Here's how the part is built. I have some questions about the finished solid (model axes, mm). A direction names the side the tool comes from. Round coordinates to 2 decimals unless told otherwise and drop trailing zeros. Write each loop counter-clockwise with the first axis right and the second up, starting at its lowest first coordinate (ties: lowest second). Pieces come first, ordered by that corner, then holes. Notation, with made-up numbers: (53.5, 57.5) - (82.5, 57.5) arc R16 cw to (82.5, 77.5) - close; hole circle Ø7 at (-30, 37). An arc over 180 degrees is marked (long way). Write item = value, one per line. Start each with the question number.
Item 1: For P1, Ø7.5, axis at x = -18.12, z = -32.26, coming from the -Y side; P2, Ø7.5, axis at x = -37, z = -0.43, coming from the +Y side, each with a flat end and sliding along its axis, tell me the tip position at first contact or that it passes through.
Item 2: If we section it at D-D (y = -17.25): Please give me the cut outline in (x, z), and give its area (3 significant figures).
Item 3: If we section it at C-C (y = -2.25): Please give me the cut outline in (x, z), and give its area (3 significant figures).
Item 4: If we section it at A-A (x = 0): Please give me the cut outline in (y, z), and give its area (3 significant figures).
Item 5: Which directions (+Z, -Z, +X, -X, +Y, -Y) give clear straight access to the entire face, cutting with the end or side of a thin tool? Please do faces 4 (the face through (-18.75, -2.46, 34.62)), 5 (the face through (-10, -15, -51)), 6 (the face through (6, 0, 32)).
Item 6: If we section it at B-B (z = 0): Please give me the cut outline in (x, y), and give its area (3 significant figures).
Item 7: Thinking about a two-plate mould opening in Z: for faces 1 (the face through (-28, -5, 16)), 2 (the face through (-2, -5, -60)), 3 (the face through (0, -10, -51)), which applies, pulls with the +Z half, pulls with the -Z half, needs draft (parallel to the pull), parting line crosses it, or undercut?
Item 8: If I drill on line 1 along X through (y, z) = (-3.7, 0); line 2 along X through (y, z) = (-12, 0); line 3 along X through (y, z) = (2.5, 0), over which ranges is the centre line in solid material (lowest first)? Write a range as [from, to].
```python
from build123d import *

# Parameters (mm, degrees)
SKETCH1_W               = 220
SKETCH1_H               = 120
SKETCH1_R               = 43
BOSS_EXTRUDE1_DEPTH     = 10
SKETCH2_W               = 220
SKETCH2_H               = 120
SKETCH2_R               = 2.8
BOSS_EXTRUDE2_DEPTH     = 20
CUT_EXTRUDE1_REACH      = 166.012
CUT_EXTRUDE1_END_RADIUS = 43
SKETCH3_W               = 35
SKETCH3_H               = 10
SKETCH4_R               = 32
CUT_EXTRUDE2_DEPTH      = 127.885775404
CUT_EXTRUDE3_REACH      = 166.012
CUT_EXTRUDE3_END_RADIUS = 32
SKETCH5_W               = 20
SKETCH5_H               = 10
SKETCH6_R               = 42.5
CUT_EXTRUDE4_DEPTH      = 15


with BuildPart() as part:
    # Sketch1 → Boss-Extrude1 (new body)
    with BuildSketch(Plane(origin=(0, 0, 0), x_dir=(1, 0, 0), z_dir=(0, 1, 0))):
        Rectangle(SKETCH1_W, SKETCH1_H)
        with Locations(Location((0, 0, 0), (0, 0, 270))):
            Circle(SKETCH1_R, mode=Mode.SUBTRACT)
    extrude(amount=BOSS_EXTRUDE1_DEPTH)

    # Sketch2 → Boss-Extrude2 (add)
    with BuildSketch(Plane.XZ):
        Rectangle(SKETCH2_W, SKETCH2_H)
        with Locations(Location((18.122136771, 32.25814872, 0), (0, 0, 270))):
            Circle(SKETCH2_R, mode=Mode.SUBTRACT)
        with Locations(Location((36.997444656, 0.434843546, 0), (0, 0, 270))):
            Circle(SKETCH2_R, mode=Mode.SUBTRACT)
        with Locations(Location((18.875307886, -31.823305174, 0), (0, 0, 270))):
            Circle(SKETCH2_R, mode=Mode.SUBTRACT)
        with Locations(Location((-18.122136771, -32.25814872, 0), (0, 0, 270))):
            Circle(SKETCH2_R, mode=Mode.SUBTRACT)
        with Locations(Location((-36.997444656, -0.434843546, 0), (0, 0, 270))):
            Circle(SKETCH2_R, mode=Mode.SUBTRACT)
        with Locations(Location((-18.875307886, 31.823305174, 0), (0, 0, 270))):
            Circle(SKETCH2_R, mode=Mode.SUBTRACT)
    extrude(amount=BOSS_EXTRUDE2_DEPTH)

    # Cut-Extrude1: up to this cylinder (the profile starts outside it)
    cut_extrude1_end = Plane(origin=(0, 5, 0), z_dir=(0, -1, 0)) * Cylinder(CUT_EXTRUDE1_END_RADIUS, 419.024, mode=Mode.PRIVATE)
    # Sketch3 → Cut-Extrude1 (cut, up to the surface)
    with BuildSketch(Plane.XY.offset(60), mode=Mode.PRIVATE) as cut_extrude1_sk1:
        with Locations((0, 5)):
            Rectangle(SKETCH3_W, SKETCH3_H)
    cut_extrude1_tool1 = extrude(cut_extrude1_sk1.sketch, amount=-CUT_EXTRUDE1_REACH, mode=Mode.PRIVATE) - cut_extrude1_end
    add(cut_extrude1_tool1.solids().sort_by_distance((0, 5, 60))[0], mode=Mode.SUBTRACT)

    # Sketch4 → Cut-Extrude2 (cut, through all)
    with BuildSketch(Plane(origin=(0, 0, 0), x_dir=(1, 0, 0), z_dir=(0, 1, 0))):
        with Locations(Location((0, 0, 0), (0, 0, 270))):
            Circle(SKETCH4_R)
    extrude(amount=-CUT_EXTRUDE2_DEPTH, mode=Mode.SUBTRACT)

    # Cut-Extrude3: up to this cylinder (the profile starts outside it)
    cut_extrude3_end = Plane(origin=(0, -15, 0), z_dir=(0, 1, 0)) * Cylinder(CUT_EXTRUDE3_END_RADIUS, 397.024, mode=Mode.PRIVATE)
    # Sketch5 → Cut-Extrude3 (cut, up to the surface)
    with BuildSketch(Plane(origin=(0, 0, -60), x_dir=(-1, 0, 0), z_dir=(0, 0, -1)), mode=Mode.PRIVATE) as cut_extrude3_sk1:
        with Locations((0, -15)):
            Rectangle(SKETCH5_W, SKETCH5_H)
    cut_extrude3_tool1 = extrude(cut_extrude3_sk1.sketch, amount=-CUT_EXTRUDE3_REACH, mode=Mode.PRIVATE) - cut_extrude3_end
    add(cut_extrude3_tool1.solids().sort_by_distance((0, -15, -60))[0], mode=Mode.SUBTRACT)

    # Sketch6 → Cut-Extrude4 (cut)
    with BuildSketch(Plane.XZ.offset(20)):
        with Locations(Location((0, 0, 0), (0, 0, 270))):
            Circle(SKETCH6_R)
    extrude(amount=-CUT_EXTRUDE4_DEPTH, mode=Mode.SUBTRACT)


solid = part.part
```
Reply:
q1.P1 = -5
q1.P2 = 0
q2.outline = (-110, -60) - (-10, -60) - (-10, -41.31) arc R42.5 cw (long way) to (10, -41.31) - (10, -60) - (110, -60) - (110, 60) - (-110, 60) - close
q2.area = 20,400 mm2
q3.outline = (-110, -60) - (110, -60) - (110, 60) - (-110, 60) - close; hole circle Ø5.6 at (-37, -0.43); hole circle Ø64 at (0, 0); hole circle Ø5.6 at (-18.88, 31.82); hole circle Ø5.6 at (-18.12, -32.26); hole circle Ø5.6 at (18.12, 32.26); hole circle Ø5.6 at (18.88, -31.82); hole circle Ø5.6 at (37, 0.43)
q3.area = 23,000 mm2
q4.outline = (-20, 42.5) - (-5, 42.5) - (-5, 32) - (0, 32) - (0, 60) - (-20, 60) - close; (-10, -60) - (10, -60) - (10, -43) - (0, -43) - (0, -32) - (-5, -32) - (-5, -42.5) - (-10, -42.5) - close
q4.area = 800 mm2
q5.face_4 = +Y, -Y
q5.face_5 = -Z, -Y
q5.face_6 = +Y
q6.outline = (-110, -20) - (-42.5, -20) - (-42.5, -5) - (-39.76, -5) - (-39.76, 0) - (-43, 0) - (-43, 10) - (-110, 10) - close; (-34.23, -5) - (-32, -5) - (-32, 0) - (-34.23, 0) - close; (32, -5) - (34.23, -5) - (34.23, 0) - (32, 0) - close; (39.76, -5) - (42.5, -5) - (42.5, -20) - (110, -20) - (110, 10) - (43, 10) - (43, 0) - (39.76, 0) - close
q6.area = 4,090 mm2
q7.face_1 = undercut
q7.face_2 = pulls with the -Z half
q7.face_3 = needs draft
q8.line_1 = [-110, -39.76], [-34.23, -32], [32, 34.23], [39.76, 110]
q8.line_2 = [-110, -42.5], [42.5, 110]
q8.line_3 = [-110, -43], [43, 110]
